from build123d import *

# Parameters (mm, degrees)
F0_W     = 40
F0_H     = 700
F1_DEPTH = 20
F3_DEPTH = 50
F5_DEPTH = 50
F6_R     = 4
F7_DEPTH = 25
F8_R     = 0.5


with BuildPart() as f1:
    # F0 (on Front) → F1 (new body)
    with BuildSketch(Plane.XZ):
        with Locations((20, 350)):
            Rectangle(F0_W, F0_H)
    extrude(amount=F1_DEPTH)

    # F2 (on face) → F3 (cut)
    with BuildSketch(Plane.XY.offset(700)):
        with BuildLine():
            ThreePointArc((20, 0), (27.071068, -2.928932), (30, -10))
            ThreePointArc((30, -10), (27.071068, -17.071068), (20, -20))
            Line((20, -20), (40, -20))
            Line((40, -20), (40, 0))
            Line((40, 0), (20, 0))
        make_face()
        with BuildLine():
            ThreePointArc((20, -20), (10, -10), (20, 0))
            Line((20, 0), (0, 0))
            Line((0, 0), (0, -20))
            Line((0, -20), (20, -20))
        make_face()
    extrude(amount=-F3_DEPTH, mode=Mode.SUBTRACT)

    # F4 (on face) → F5 (cut)
    with BuildSketch(Plane(origin=(0, 0, 0), x_dir=(1, 0, 0), z_dir=(0, 0, -1))):
        with BuildLine():
            ThreePointArc((20, 0), (10, 10), (20, 20))
            Line((20, 20), (0, 20))
            Line((0, 20), (0, 0))
            Line((0, 0), (20, 0))
        make_face()
        with BuildLine():
            ThreePointArc((20, 20), (27.071068, 17.071068), (30, 10))
            ThreePointArc((30, 10), (27.071068, 2.928932), (20, 0))
            Line((20, 0), (40, 0))
            Line((40, 0), (40, 20))
            Line((40, 20), (20, 20))
        make_face()
    extrude(amount=-F5_DEPTH, mode=Mode.SUBTRACT)

    # F6 (on face) → F7 (cut)
    with BuildSketch(Plane(origin=(0, 0, 0), x_dir=(-1, 0, 0), z_dir=(0, 1, 0))):
        with Locations((-20, 470)):
            Circle(F6_R)
        with Locations((-20, 230)):
            Circle(F6_R)
        with Locations((-20, 350)):
            Circle(F6_R)
    extrude(amount=-F7_DEPTH, mode=Mode.SUBTRACT)

    # F8
    f8_edges = [f1.edges().sort_by_distance(p)[0] for p in [
        (0, 0, 350),
        (0, -20, 350),
        (40, 0, 350),
        (40, -20, 350),
    ]]
    fillet(f8_edges, radius=F8_R)


solid = f1.part
Read the model definition and answer for the solid it produces. Units are mm, in the model's axes. A direction names the side the tool comes from. Coordinates: 2 decimals unless noted, no trailing zeros. Loops run counter-clockwise (first coordinate to the right, second up) from the corner with the lowest first, then second, coordinate; pieces in that order, holes last.
Q1. This flat-tipped pin is pushed along its axis until it touches: pin 1 Ø8 at (x, y) = (5.5, -4.5) entering from +Z. Where does it stop, or does it pass through?
Q2. The part is cut by section A-A on y = -14.5. Write down the section's boundary in (x, z), and give its area (3 significant figures).
Q3. Consider probe 1 along Z at (x, y) = (20, -15.25); probe 2 along Z at (x, y) = (19, -10.5); probe 3 along X at (y, z) = (-5.5, 470). Determine where each line is inside the solid, lowest interval first.
Q4. Which of the six approach directions +Z, -Z, +X, -X, +Y, -Y give full straight-line access (tool end or side, diameter ignored) to faces 1 (the face through (20, -10, 0)), 2 (the face through (34, -10, 50)), 3 (the face through (34, -10, 650))?
Results below:
1. pin 1: stops at z = 650
2. outline: (0, 50) - (11.07, 50) - (11.07, 0) - (28.93, 0) - (28.93, 50) - (40, 50) - (40, 650) - (28.93, 650) - (28.93, 700) - (11.07, 700) - (11.07, 650) - (0, 650) - close; hole circle Ø8 at (20, 230); hole circle Ø8 at (20, 350); hole circle Ø8 at (20, 470)
2. area: 25,600 mm2
3. probe 1: z = 0 to 226, 234 to 346, 354 to 466, 474 to 700
3. probe 2: z = 0 to 226.13, 233.87 to 346.13, 353.87 to 466.13, 473.87 to 700
3. probe 3: x = 0 to 16, 24 to 40
4. face 1: -Z, +X, -X, +Y, -Y
4. face 2: -Z, +X
4. face 3: +Z, +X
